from build123d import *

# Parameters (mm, degrees)
EXTRUDE_1_DEPTH     = 6
SKETCH_2_W          = 56.5
SKETCH_2_H          = 56.5
CUT_EXTRUDE_1_DEPTH = 3
CUT_EXTRUDE_2_DEPTH = 6


with BuildPart() as part:
    # 草图1 → 凸台-拉伸1 (new body)
    with BuildSketch(Plane.XY):
        Polygon((22.5, 0), (62.5, 0), (62.5, 27.144660941), (147.352813742, 111.997474683), (111.997474683, 147.352813742), (27.144660941, 62.5), (0, 62.5), (0, 22.5), (6, 22.5), (6, 56.5), (56.5, 56.5), (56.5, 6), (22.5, 6), align=None)
    extrude(amount=EXTRUDE_1_DEPTH)

    # 草图2 → 切除-拉伸1 (cut)
    with BuildSketch(Plane.XY.offset(6)):
        with Locations((31.156538063, 31.156538063)):
            Rectangle(SKETCH_2_W, SKETCH_2_H)
    extrude(amount=-CUT_EXTRUDE_1_DEPTH, mode=Mode.SUBTRACT)

    # 草图3 → 切除-拉伸2 (cut)
    with BuildSketch(Plane.XY.offset(6)):
        with BuildLine():
            Line((112.88135816, 127.023493783), (127.023493783, 112.88135816))
            ThreePointArc((127.023493783, 112.88135816), (129.498367517, 112.88135816), (129.498367517, 115.356231894))
            Line((129.498367517, 115.356231894), (115.356231894, 129.498367517))
            ThreePointArc((115.356231894, 129.498367517), (112.88135816, 129.498367517), (112.88135816, 127.023493783))
        make_face()
    extrude(amount=-CUT_EXTRUDE_2_DEPTH, mode=Mode.SUBTRACT)


solid = part.part
Build history of the part. All positions in model axes, mm. A direction names the side the tool comes from. Round coordinates to 2 decimals unless told otherwise and drop trailing zeros. Loops run counter-clockwise (first coordinate to the right, second up) from the corner with the lowest first, then second, coordinate; pieces in that order, holes last. Notation, with made-up numbers: (83, 32) -> (92, 32) arc R37 cw to (92, 71) -> close; hole circle Ø4 at (-13, 48.5). An arc over 180 degrees is marked (long way). Use CSV: the item, a comma, the result in double quotes. Start each with the question number.
Q1. Saw through at D-D on x = 14. Give the cut face in (y, z), and give its area (3 significant figures).
Q2. Which spindle directions (+Z, -Z, +X, -X, +Y, -Y) get a long thin tool onto all of the face, cutting with end or side? Do faces 4 (the face through (119.853, 120.051, 3.042)), 5 (the face through (14, 62.5, 3)), 6 (the face through (2, 22.5, 2)). Say none if no direction does.
Q3. Drill centre lines: L1, parallel to Y at x = 24, z = 1.4; L2, parallel to X at y = 26, z = 5.4; L3, parallel to Y at x = 45, z = 1.2. Where is each one in solid material? Low to high.
Q4. Saw through at A-A on z = 4.85. Give the cut face in (x, y).
Q5. Mould opens along X. For faces 1 (the face through (31, 58, 3)), 2 (the face through (62.5, 13, 3)), 3 (the face through (22.5, 2, 2)) say: +X half, -X half, draft (parallel to the pull), parting line (faces both ways), or undercut.
Q6. Saw through at B-B on y = 32.5. Give the cut face in (x, z), and give its area (3 significant figures).
Q7. Saw through at C-C on x = 50. Give the cut face in (y, z), and give its area (3 significant figures).
Q8. Flat gauge pins, fed straight in: pin 1 Ø0.9 at (y, z) = (19, 1) entering from -X; pin 2 Ø1.5 at (y, z) = (40, 1) entering from +X; pin 3 Ø1.5 at (y, z) = (17, 4.5) entering from -X. Where does each tip first touch, or does it go through?
Solutions:
1,outline,"(56.5, 0) -> (62.5, 0) -> (62.5, 6) -> (59.41, 6) -> (59.41, 3) -> (56.5, 3) -> close"
1,area,"27.3 mm^2"
2,face 4,"+Z, -Z"
2,face 5,"+Z, -Z, -X, +Y"
2,face 6,"+Z, -Z, -X, -Y"
3,L1,"y = 0 to 6, 56.5 to 62.5"
3,L2,"x = 0 to 2.91, 59.41 to 62.5"
3,L3,"y = 0 to 6, 56.5 to 80.36"
4,outline,"(0, 22.5) -> (2.91, 22.5) -> (2.91, 59.41) -> (59.41, 59.41) -> (59.41, 2.91) -> (22.5, 2.91) -> (22.5, 0) -> (62.5, 0) -> (62.5, 27.14) -> (147.35, 112) -> (112, 147.35) -> (27.14, 62.5) -> (0, 62.5) -> close; hole (112.88, 127.02) -> (127.02, 112.88) arc R1.75 ccw to (129.5, 115.36) -> (115.36, 129.5) arc R1.75 ccw to start"
5,face 1,"undercut"
5,face 2,"+X half"
5,face 3,"-X half"
6,outline,"(0, 0) -> (6, 0) -> (6, 3) -> (2.91, 3) -> (2.91, 6) -> (0, 6) -> close; (56.5, 0) -> (67.86, 0) -> (67.86, 6) -> (59.41, 6) -> (59.41, 3) -> (56.5, 3) -> close"
6,area,"86.1 mm^2"
7,outline,"(0, 0) -> (6, 0) -> (6, 3) -> (2.91, 3) -> (2.91, 6) -> (0, 6) -> close; (56.5, 0) -> (85.36, 0) -> (85.36, 6) -> (59.41, 6) -> (59.41, 3) -> (56.5, 3) -> close"
7,area,"191 mm^2"
8,pin 1,"stops at x = 56.5"
8,pin 2,"stops at x = 76.11"
8,pin 3,"stops at x = 59.41"
